Source: CAD feature listing. Evaluate the final solid. Frame: model axes, mm. A direction names the side the tool comes from. Round coordinates to 2 decimals unless told otherwise and drop trailing zeros. Loops run counter-clockwise (first coordinate to the right, second up) from the corner with the lowest first, then second, coordinate; pieces in that order, holes last. Notation, with made-up numbers: (-38.5, 14) - (19.5, 14) arc R26 cw to (19.5, 38) - close; hole circle Ø9 at (19.25, 73). An arc over 180 degrees is marked (long way). One line per question, with ' | ' between items.
from build123d import *

# Parameters (mm, degrees)
F0_W      = 76.2
F0_H      = 76.2
F1_DEPTH  = 76.2
F2_R      = 7.62
F3_R      = 6.3632045514
F4_DEPTH  = 5.08
F6_DEPTH  = 5.08
F7_DEPTH  = 5.08
F9_R      = 6.35
F10_DEPTH = 5.08
F11_R     = 6.35
F12_DEPTH = 5.08
F13_R     = 6.35
F14_DEPTH = 5.08
F15_R     = 6.35
F16_DEPTH = 5.08


with BuildPart() as f1:
    # F0 (on Top) → F1 (new body)
    with BuildSketch(Plane.XY):
        with Locations((-8.1155080592, -6.2860166654)):
            Rectangle(F0_W, F0_H)
    extrude(amount=F1_DEPTH)

    # F2
    f2_edges = [f1.edges().sort_by_distance(p)[0] for p in [
        (-46.215508, 31.813983, 38.1),
        (29.984492, 31.813983, 38.1),
        (29.984492, -44.386017, 38.1),
        (-46.215508, -44.386017, 38.1),
        (-8.115508, 31.813983, 0),
        (-8.115508, 31.813983, 76.2),
        (-8.115508, -44.386017, 0),
        (-8.115508, -44.386017, 76.2),
        (29.984492, -6.286017, 0),
        (29.984492, -6.286017, 76.2),
        (-46.215508, -6.286017, 0),
        (-46.215508, -6.286017, 76.2),
    ]]
    fillet(f2_edges, radius=F2_R)

    # F3 (on face) → F4 (cut)
    with BuildSketch(Plane.XY.offset(76.2)):
        with Locations((-8.1155080592, -6.2860166654)):
            Circle(F3_R)
    extrude(amount=-F4_DEPTH, mode=Mode.SUBTRACT)

    # F5 (on face) → F6 (cut)
    with BuildSketch(Plane(origin=(0, 0, 0), x_dir=(1, 0, 0), z_dir=(0, 0, -1))):
        with BuildLine():
            ThreePointArc((-17.7270988166, 6.2860166654), (-19.5869707561, 10.7761447259), (-24.0770988166, 12.6360166654))
            Line((-24.0770988166, 12.6360166654), (-24.0770988166, -0.0639833346))
            ThreePointArc((-24.0770988166, -0.0639833346), (-19.5869707561, 1.7958886049), (-17.7270988166, 6.2860166654))
        make_face()
        with BuildLine():
            Line((-24.0770988166, -0.0639833346), (-24.0770988166, 12.6360166654))
            ThreePointArc((-24.0770988166, 12.6360166654), (-30.4270988166, 6.2860166654), (-24.0770988166, -0.0639833346))
        make_face()
        with BuildLine():
            ThreePointArc((14.8022180259, 25.3360166654), (12.9423460865, 29.8261447259), (8.4522180259, 31.6860166654))
            Line((8.4522180259, 31.6860166654), (8.4522180259, 18.9860166654))
            ThreePointArc((8.4522180259, 18.9860166654), (12.9423460865, 20.8458886049), (14.8022180259, 25.3360166654))
        make_face()
        with BuildLine():
            Line((8.4522180259, 18.9860166654), (8.4522180259, 31.6860166654))
            ThreePointArc((8.4522180259, 31.6860166654), (2.1022180259, 25.3360166654), (8.4522180259, 18.9860166654))
        make_face()
        with BuildLine():
            Line((8.4522180259, -0.0639833346), (8.4522180259, 12.6360166654))
            ThreePointArc((8.4522180259, 12.6360166654), (2.1022180259, 6.2860166654), (8.4522180259, -0.0639833346))
        make_face()
        with BuildLine():
            ThreePointArc((14.8022180259, 6.2860166654), (12.9423460865, 10.7761447259), (8.4522180259, 12.6360166654))
            Line((8.4522180259, 12.6360166654), (8.4522180259, -0.0639833346))
            ThreePointArc((8.4522180259, -0.0639833346), (12.9423460865, 1.7958886049), (14.8022180259, 6.2860166654))
        make_face()
        with BuildLine():
            Line((-24.0770988166, 18.9860166654), (-24.0770988166, 31.6860166654))
            ThreePointArc((-24.0770988166, 31.6860166654), (-30.4270988166, 25.3360166654), (-24.0770988166, 18.9860166654))
        make_face()
        with BuildLine():
            ThreePointArc((8.4522180259, -6.4139833346), (2.1022180259, -12.7639833346), (8.4522180259, -19.1139833346))
            Line((8.4522180259, -19.1139833346), (8.4522180259, -6.4139833346))
        make_face()
        with BuildLine():
            Line((8.4522180259, -6.4139833346), (8.4522180259, -19.1139833346))
            ThreePointArc((8.4522180259, -19.1139833346), (12.9423460865, -17.2541113951), (14.8022180259, -12.7639833346))
            ThreePointArc((14.8022180259, -12.7639833346), (12.9423460865, -8.2738552741), (8.4522180259, -6.4139833346))
        make_face()
        with BuildLine():
            Line((-24.0770988166, -6.4139833346), (-24.0770988166, -19.1139833346))
            ThreePointArc((-24.0770988166, -19.1139833346), (-19.5869707561, -17.2541113951), (-17.7270988166, -12.7639833346))
            ThreePointArc((-17.7270988166, -12.7639833346), (-19.5869707561, -8.2738552741), (-24.0770988166, -6.4139833346))
        make_face()
        with BuildLine():
            ThreePointArc((-24.0770988166, -6.4139833346), (-30.4270988166, -12.7639833346), (-24.0770988166, -19.1139833346))
            Line((-24.0770988166, -19.1139833346), (-24.0770988166, -6.4139833346))
        make_face()
        with BuildLine():
            ThreePointArc((-17.7270988166, 25.3360166654), (-19.5869707561, 29.8261447259), (-24.0770988166, 31.6860166654))
            Line((-24.0770988166, 31.6860166654), (-24.0770988166, 18.9860166654))
            ThreePointArc((-24.0770988166, 18.9860166654), (-19.5869707561, 20.8458886049), (-17.7270988166, 25.3360166654))
        make_face()
    extrude(amount=-F6_DEPTH, mode=Mode.SUBTRACT)

    # F7 (add): a face of the model
    f7_faces = [f1.faces().sort_by_distance(p)[0] for p in [
        (-46.2155080592, -6.2860166654, 38.1),
    ]]
    extrude(f7_faces, amount=-F7_DEPTH)

    # F9 (on face) → F10 (cut)
    with BuildSketch(Plane(origin=(-46.2155080592, 0, 0), x_dir=(0, -1, 0), z_dir=(-1, 0, 0))):
        with Locations((-8.8818371296, 53.34)):
            Circle(F9_R)
        with Locations((21.0777521133, 22.86)):
            Circle(F9_R)
    extrude(amount=-F10_DEPTH, mode=Mode.SUBTRACT)

    # F11 (on face) → F12 (cut)
    with BuildSketch(Plane.YZ.offset(29.9844919408)):
        with Locations((-21.9498630613, 53.34)):
            Circle(F11_R)
        with BuildLine():
            ThreePointArc((0.0639833346, 38.1), (-1.7958886049, 42.5901280605), (-6.2860166654, 44.45))
            Line((-6.2860166654, 44.45), (-6.2860166654, 38.1))
            Line((-6.2860166654, 38.1), (0.0639833346, 38.1))
        make_face()
        with BuildLine():
            ThreePointArc((-6.2860166654, 31.75), (-1.7958886049, 33.6098719395), (0.0639833346, 38.1))
            Line((0.0639833346, 38.1), (-6.2860166654, 38.1))
            Line((-6.2860166654, 38.1), (-6.2860166654, 31.75))
        make_face()
        with BuildLine():
            Line((-6.2860166654, 31.75), (-6.2860166654, 38.1))
            Line((-6.2860166654, 38.1), (-12.6360166654, 38.1))
            ThreePointArc((-12.6360166654, 38.1), (-10.7761447259, 33.6098719395), (-6.2860166654, 31.75))
        make_face()
        with BuildLine():
            Line((-6.2860166654, 38.1), (-6.2860166654, 44.45))
            ThreePointArc((-6.2860166654, 44.45), (-10.7761447259, 42.5901280605), (-12.6360166654, 38.1))
            Line((-12.6360166654, 38.1), (-6.2860166654, 38.1))
        make_face()
        with Locations((8.8817877695, 53.34)):
            Circle(F11_R)
        with Locations((9.5079327002, 22.86)):
            Circle(F11_R)
        with Locations((-21.9527687877, 22.86)):
            Circle(F11_R)
    extrude(amount=-F12_DEPTH, mode=Mode.SUBTRACT)

    # F13 (on face) → F14 (cut)
    with BuildSketch(Plane.XZ.offset(44.3860166654)):
        with Locations((-24.1356771439, 53.34)):
            Circle(F13_R)
        with BuildLine():
            ThreePointArc((-1.7655080592, 38.1), (-3.6253799987, 42.5901280605), (-8.1155080592, 44.45))
            Line((-8.1155080592, 44.45), (-8.1155080592, 38.1))
            Line((-8.1155080592, 38.1), (-1.7655080592, 38.1))
        make_face()
        with BuildLine():
            ThreePointArc((-8.1155080592, 31.75), (-3.6253799987, 33.6098719395), (-1.7655080592, 38.1))
            Line((-1.7655080592, 38.1), (-8.1155080592, 38.1))
            Line((-8.1155080592, 38.1), (-8.1155080592, 31.75))
        make_face()
        with BuildLine():
            Line((-8.1155080592, 31.75), (-8.1155080592, 38.1))
            Line((-8.1155080592, 38.1), (-14.4655080592, 38.1))
            ThreePointArc((-14.4655080592, 38.1), (-12.6056361198, 33.6098719395), (-8.1155080592, 31.75))
        make_face()
        with BuildLine():
            Line((-8.1155080592, 38.1), (-8.1155080592, 44.45))
            ThreePointArc((-8.1155080592, 44.45), (-12.6056361198, 42.5901280605), (-14.4655080592, 38.1))
            Line((-14.4655080592, 38.1), (-8.1155080592, 38.1))
        make_face()
        with Locations((7.0330761373, 22.86)):
            Circle(F13_R)
    extrude(amount=-F14_DEPTH, mode=Mode.SUBTRACT)

    # F15 (on face) → F16 (cut)
    with BuildSketch(Plane(origin=(0, 31.8139833346, 0), x_dir=(-1, 0, 0), z_dir=(0, 1, 0))):
        with Locations((24.0265242755, 22.86)):
            Circle(F15_R)
        with Locations((24.1574160755, 53.34)):
            Circle(F15_R)
        with Locations((-6.5224412829, 53.34)):
            Circle(F15_R)
        with Locations((-7.0802713744, 22.86)):
            Circle(F15_R)
    extrude(amount=-F16_DEPTH, mode=Mode.SUBTRACT)


solid = f1.part
1. Mould query, pull axis Z, two halves, no side actions, for faces 1 (the cylindrical face through (-7.69, -42.21, 2.29)), 2 (the flat face through (-46.216, -7, 38)), 3 (the cylindrical face through (27.48, -26.99, 49.48)). Classes: released by +Z, released by -Z, zero draft, split by the parting line, or undercut.
Worked out:
face 1: released by -Z | face 2: zero draft | face 3: undercut
2. Section query D-D, the plane x = -11.5. Return loops of the section in (y, z), plus the area to 3 significant figures.
Worked out:
outline: (-44.39, 7.62) arc R7.62 ccw to (-36.77, 0) - (24.19, 0) arc R7.62 ccw to (31.81, 7.62) - (31.81, 68.58) arc R7.62 ccw to (24.19, 76.2) - (-0.9, 76.2) - (-0.9, 71.12) - (-11.67, 71.12) - (-11.67, 76.2) - (-36.77, 76.2) arc R7.62 ccw to (-44.39, 68.58) - (-44.39, 43.47) - (-39.31, 43.47) - (-39.31, 32.73) - (-44.39, 32.73) - close | area: 5,650 mm2
3. Section query C-C, the plane y = 17. Return loops of the section in (x, z), plus the area to 3 significant figures.
Worked out:
outline: (-46.22, 7.62) arc R7.62 ccw to (-38.6, 0) - (-28.81, 0) - (-28.81, 5.08) - (-19.35, 5.08) - (-19.35, 0) - (3.72, 0) - (3.72, 5.08) - (13.18, 5.08) - (13.18, 0) - (22.36, 0) arc R7.62 ccw to (29.98, 7.62) - (29.98, 68.58) arc R7.62 ccw to (22.36, 76.2) - (-38.6, 76.2) arc R7.62 ccw to (-46.22, 68.58) - close | area: 5,660 mm2
4. Access query for faces 4 (the cylindrical face through (-19.1, 29.3, 49.5)), 5 (the flat face through (-8, -6, 71.12)), 6 (the flat face through (-24, -25, 5.08)), 7 (the cylindrical face through (-43.711, 13.921, 49.476)), 8 (the cylindrical face through (27.48, -15.896, 24.767)). Directions: +Z, -Z, +X, -X, +Y, -Y. A direction counts if a zero-diameter tool reaches every point of the face in a straight line with its end or side. Return the directions, or none.
Worked out:
face 4: +Y | face 5: +Z | face 6: -Z | face 7: -X | face 8: +X
5. Contact query for flat-ended pins moving along their axis: P1, Ø6.5, axis at x = -7.5, z = 40.5, coming from the -Y side; P2, Ø10, axis at y = 9.51, z = 22.86, coming from the +X side; P3, Ø7.5, axis at x = -24.14, z = 53.34, coming from the +Y side. Output: stop coordinate, or through.
Worked out:
P1: stops at y = -39.31 | P2: stops at x = 24.9 | P3: stops at y = 26.73
6. Material intervals for probe 1 along Y at (x, z) = (-23, 54); probe 2 along X at (y, z) = (28, 53); probe 3 along X at (y, z) = (29, 53), sorted ascending.
Worked out:
probe 1: y = -39.31 to 26.73 | probe 2: x = -45.2 to -30.5, -17.82 to 0.18, 12.86 to 28.97 | probe 3: x = -44.51 to -30.5, -17.82 to 0.18, 12.86 to 28.28
